Here's how the part is built. I have some questions about the finished solid (model axes, mm). A direction names the side the tool comes from. Give positions to 0.01 mm unless a question says otherwise; leave off trailing zeros. Loops run counter-clockwise (first coordinate to the right, second up) from the corner with the lowest first, then second, coordinate; pieces in that order, holes last. Notation, with made-up numbers: (20, -3.5) - (25, -3.5) arc R17 cw to (25, 7.5) - close; hole circle Ø5 at (25, 70). An arc over 180 degrees is marked (long way). Use one line per item in the form item = value.
from build123d import *

# Parameters (mm, degrees)
DODANIE_WYCI_GNI_CIE1_DEPTH      = 20
DODANIE_WYCI_GNI_CIE1_DEPTH_BACK = 20
DODANIE_WYCI_GNI_CIE2_DEPTH      = 20
DODANIE_WYCI_GNI_CIE2_DEPTH_BACK = 20
DODANIE_WYCI_GNI_CIE3_DEPTH      = 20
DODANIE_WYCI_GNI_CIE3_DEPTH_BACK = 20
DODANIE_WYCI_GNI_CIE4_DEPTH      = 20
DODANIE_WYCI_GNI_CIE4_DEPTH_BACK = 20


with BuildPart() as part:
    # Szkic4 → Dodanie-wyci_gni_cie1 (new body, two sides)
    with BuildSketch(Plane(origin=(179.528354859, 0, -336.615665361), x_dir=(0.882352941, 0, 0.470588235), z_dir=(-0.470588235, 0, 0.882352941))) as dodanie_wyci_gni_cie1_sk:
        Polygon((-984.691711107, 436.10738255), (529.057535882, -283.89261745), (715.308288893, -283.89261745), (-798.440958097, 436.10738255), align=None)
    extrude(amount=DODANIE_WYCI_GNI_CIE1_DEPTH)
    extrude(dodanie_wyci_gni_cie1_sk.sketch, amount=-DODANIE_WYCI_GNI_CIE1_DEPTH_BACK)

    # Szkic5 → Dodanie-wyci_gni_cie2 (add, two sides)
    with BuildSketch(Plane(origin=(179.528354859, 0, -336.615665361), x_dir=(0.882352941, 0, 0.470588235), z_dir=(-0.470588235, 0, 0.882352941))) as dodanie_wyci_gni_cie2_sk:
        Polygon((-984.691711107, -283.89261745), (529.057535882, 436.10738255), (715.308288893, 436.10738255), (-798.440958097, -283.89261745), align=None)
    extrude(amount=DODANIE_WYCI_GNI_CIE2_DEPTH)
    extrude(dodanie_wyci_gni_cie2_sk.sketch, amount=-DODANIE_WYCI_GNI_CIE2_DEPTH_BACK)

    # Szkic6 → Dodanie-wyci_gni_cie3 (add, two sides)
    with BuildSketch(Plane(origin=(-152.651575936, 0, -286.221704881), x_dir=(0.882352941, 0, -0.470588235), z_dir=(0.470588235, 0, 0.882352941))) as dodanie_wyci_gni_cie3_sk:
        Polygon((1091.778877128, -283.89261745), (-421.970369861, 436.10738255), (-608.221122872, 436.10738255), (905.528124117, -283.89261745), align=None)
    extrude(amount=DODANIE_WYCI_GNI_CIE3_DEPTH)
    extrude(dodanie_wyci_gni_cie3_sk.sketch, amount=-DODANIE_WYCI_GNI_CIE3_DEPTH_BACK)

    # Szkic7 → Dodanie-wyci_gni_cie4 (add, two sides)
    with BuildSketch(Plane(origin=(-152.651575936, 0, -286.221704881), x_dir=(0.882352941, 0, -0.470588235), z_dir=(0.470588235, 0, 0.882352941))) as dodanie_wyci_gni_cie4_sk:
        Polygon((-421.970369861, -283.89261745), (1091.778877128, 436.10738255), (905.528124117, 436.10738255), (-608.221122872, -283.89261745), align=None)
    extrude(amount=DODANIE_WYCI_GNI_CIE4_DEPTH)
    extrude(dodanie_wyci_gni_cie4_sk.sketch, amount=-DODANIE_WYCI_GNI_CIE4_DEPTH_BACK)


solid = part.part
(1) If we section it at A-A (y = -44): List the corners of the cut face in (x, z) for me.
Geometry says:
outline = (-253.71, -545.01) - (-234.88, -580.3) - (-70.55, -492.66) - (-89.37, -457.36) - close; (-253.71, -254.99) - (-89.37, -342.64) - (-70.55, -307.34) - (-234.88, -219.7) - close; (191.91, -492.66) - (356.25, -580.3) - (375.07, -545.01) - (210.73, -457.36) - close; (191.91, -307.34) - (210.73, -342.64) - (375.07, -254.99) - (356.25, -219.7) - close
(2) If we section it at B-B (x = 213): List the corners of the cut face in (y, z) for me, plus the area to 3 significant figures.
Geometry says:
outline = (-55.37, -503.9) - (33.22, -503.9) - (43.37, -458.57) - (-45.22, -458.57) - close; (-55.37, -296.1) - (-45.22, -341.43) - (43.37, -341.43) - (33.22, -296.1) - close; (108.85, -458.57) - (118.99, -503.9) - (207.58, -503.9) - (197.44, -458.57) - close; (108.85, -341.43) - (197.44, -341.43) - (207.58, -296.1) - (118.99, -296.1) - close
area = 16,100 mm²
(3) Thinking about a two-plate mould opening in X: for faces 1 (the flat face through (-360.21, 258.63, -624.16)), 2 (the flat face through (-228.18, 276.045, -246.257)), 3 (the flat face through (727, -283.893, -755)), which applies, pulls with the +X half, pulls with the -X half, needs draft (parallel to the pull), parting line crosses it, or undercut?
Geometry says:
face_1 = pulls with the -X half
face_2 = undercut
face_3 = needs draft
(4) If I drill on probe 1 along Z at (x, y) = (-226, 208); probe 2 along X at (y, z) = (-173.5, -703.5); probe 3 along X at (y, z) = (-188.5, -168), over which ranges is the centre line in solid material (lowest first)?
Geometry says:
probe_1 = -575.56 to -530.23, -269.77 to -224.44
probe_2 = -477.75 to -465.88, 587.25 to 599.11
probe_3 = -416.82 to -340.54, 461.9 to 538.18
(5) For faces 4 (the flat face through (-236.12, -128.25, -241.39)), 5 (the flat face through (-258.94, 211.12, -547.8)), 6 (the flat face through (-201.62, 184.45, -237.44)), which set-ups out of +Z, -Z, +X, -X, +Y, -Y let a thin tool reach every point of the face, with its end or its side?
Geometry says:
face_4 = -Y
face_5 = -X, +Y, -Y
face_6 = +Z, +Y, -Y
(6) For P1, Ø12, axis at y = 196, z = -559.5, coming from the -X side; P2, Ø12, axis at y = 180, z = -487.5, coming from the -X side, each with a flat end and sliding along its axis, tell me the tip position at first contact or that it passes through.
Geometry says:
P1 = -260.12
P2 = -157.13
